The listing builds one solid part. Answer for the finished solid, in the listing's coordinates (mm). A direction names the side the tool comes from. Give positions to 0.01 mm unless a question says otherwise; leave off trailing zeros. Order: outer loops, then holes, each group sorted by start corner. A loop starts at its lowest first (then second) coordinate and runs counter-clockwise, first axis right, second up. Notation, with made-up numbers: (-25.75, 42) - (-18.75, 42) arc R12 ccw to (-18.75, 65) - close; hole circle Ø1 at (35.25, 12). An arc over 180 degrees is marked (long way). Answer in a Markdown table with one row per item. Add a question column.
```python
from build123d import *

# Parameters (mm, degrees)
BOSS_EXTRUDE1_DEPTH     = 300
SKETCH2_W               = 10
SKETCH2_H               = 10
BOSS_EXTRUDE2_DEPTH     = 2
SKETCH4_R               = 18
SKETCH4_R_2             = 15
SKETCH4_R_3             = 10
BOSS_EXTRUDE3_DEPTH     = 2
SKETCH4_3_R             = 10
CUT_EXTRUDE1_DEPTH      = 2
BOSS_EXTRUDE4_START     = -5
BOSS_EXTRUDE4_OUTLINE_R = 12.5
BOSS_EXTRUDE4_DEPTH     = 3
CUT_EXTRUDE2_START      = -2
CUT_EXTRUDE2_DEPTH      = 2
F_3_0MM_DOWEL_HOLE1_D   = 3
SKETCH8_R               = 2.5
BOSS_EXTRUDE5_DEPTH     = 2
SKETCH9_R               = 5
CUT_EXTRUDE3_DEPTH      = 32
SKETCH10_R              = 2.5
CUT_EXTRUDE4_DEPTH      = 10


# Read off the part's stored shape, not the designer's step: Boss-Extrude4, Cut-Extrude2
with BuildPart() as part:
    # Sketch1 → Boss-Extrude1 (new body)
    with BuildSketch(Plane(origin=(0, 0, 0), x_dir=(0, 0, -1), z_dir=(1, 0, 0))):
        with BuildLine():
            Line((10, 13), (10, -13))
            ThreePointArc((10, -13), (9.414213562, -14.414213562), (8, -15))
            Line((8, -15), (0, -15))
            Line((0, -15), (0, -14))
            Line((0, -14), (7, -14))
            ThreePointArc((7, -14), (8.414213562, -13.414213562), (9, -12))
            Line((9, -12), (9, 12))
            ThreePointArc((9, 12), (8.414213562, 13.414213562), (7, 14))
            Line((7, 14), (0, 14))
            Line((0, 14), (0, 15))
            Line((0, 15), (8, 15))
            ThreePointArc((8, 15), (9.414213562, 14.414213562), (10, 13))
        make_face()
    extrude(amount=BOSS_EXTRUDE1_DEPTH)

    # Sketch2 → Boss-Extrude2 (add)
    with BuildSketch(Plane.XY):
        with Locations((75, 20)):
            Rectangle(SKETCH2_W, SKETCH2_H)
        with Locations((75, -20)):
            Rectangle(SKETCH2_W, SKETCH2_H)
        with Locations((225, 20)):
            Rectangle(SKETCH2_W, SKETCH2_H)
        with Locations((225, -20)):
            Rectangle(SKETCH2_W, SKETCH2_H)
    extrude(amount=-BOSS_EXTRUDE2_DEPTH)

    # Sketch4 → Boss-Extrude3 (add)
    # profile 1 of 2: a face of its own
    with BuildSketch(Plane(origin=(0, 0, -10), x_dir=(-1, 0, 0), z_dir=(0, 0, -1))):
        Circle(SKETCH4_R)
        Circle(SKETCH4_R_2, mode=Mode.SUBTRACT)
    # profile 2 of 2: a face of its own
    with BuildSketch(Plane(origin=(0, 0, -10), x_dir=(-1, 0, 0), z_dir=(0, 0, -1))):
        Circle(SKETCH4_R)
        with Locations(Location((0, 0, 0), (0, 0, 90))):
            Circle(SKETCH4_R_3, mode=Mode.SUBTRACT)
    extrude(amount=-BOSS_EXTRUDE3_DEPTH)

    # Sketch4<3> → Cut-Extrude1 (cut)
    with BuildSketch(Plane(origin=(0, 0, -10), x_dir=(-1, 0, 0), z_dir=(0, 0, -1))):
        with Locations(Location((0, 0, 0), (0, 0, 90))):
            Circle(SKETCH4_3_R)
    extrude(amount=-CUT_EXTRUDE1_DEPTH, mode=Mode.SUBTRACT)

    # Boss-Extrude4 outline → Boss-Extrude4 (add)
    with BuildSketch(Plane(origin=(0, 0, -10), x_dir=(-1, 0, 0), z_dir=(0, 0, -1)).offset(BOSS_EXTRUDE4_START)):
        Circle(BOSS_EXTRUDE4_OUTLINE_R)
        with BuildLine():
            ThreePointArc((-9.682458366, 2.5), (10, 0), (-9.682458366, -2.5))
            Line((-9.682458366, -2.5), (-10.25, -2.5))
            ThreePointArc((-10.25, -2.5), (-11.664213562, -1.914213562), (-12.25, -0.5))
            Line((-12.25, -0.5), (-12.25, 0.5))
            ThreePointArc((-12.25, 0.5), (-11.664213562, 1.914213562), (-10.25, 2.5))
            Line((-10.25, 2.5), (-9.682458366, 2.5))
        make_face(mode=Mode.SUBTRACT)
    extrude(amount=BOSS_EXTRUDE4_DEPTH)

    # Cut-Extrude2 outline → Cut-Extrude2 (cut)
    with BuildSketch(Plane(origin=(0, 0, -10), x_dir=(-1, 0, 0), z_dir=(0, 0, -1)).offset(CUT_EXTRUDE2_START)):
        with BuildLine():
            ThreePointArc((-10.25, 2.5), (-11.664213562, 1.914213562), (-12.25, 0.5))
            Line((-12.25, 0.5), (-12.25, -0.5))
            ThreePointArc((-12.25, -0.5), (-11.664213562, -1.914213562), (-10.25, -2.5))
            Line((-10.25, -2.5), (-9.682458366, -2.5))
            ThreePointArc((-9.682458366, -2.5), (-10, 0), (-9.682458366, 2.5))
            Line((-9.682458366, 2.5), (-10.25, 2.5))
        make_face()
    extrude(amount=CUT_EXTRUDE2_DEPTH, mode=Mode.SUBTRACT)

    # Ø3.0mm Dowel Hole1 (through all)
    with Locations(Plane.XY):
        with Locations((75, 20), (75, -20), (225, 20), (225, -20)):
            Hole(F_3_0MM_DOWEL_HOLE1_D / 2)

    # Sketch8 → Boss-Extrude5 (add)
    with BuildSketch(Plane(origin=(300, 0, 0), x_dir=(0, 0, -1), z_dir=(1, 0, 0))):
        with BuildLine():
            Line((0, -5), (0, -20))
            Line((0, -20), (30, -20))
            Line((30, -20), (30, 20))
            Line((30, 20), (0, 20))
            Line((0, 20), (0, 5))
            ThreePointArc((0, 5), (3.535533906, 3.535533906), (5, 0))
            ThreePointArc((5, 0), (3.535533906, -3.535533906), (0, -5))
        make_face()
        with Locations((23, -13)):
            Circle(SKETCH8_R, mode=Mode.SUBTRACT)
        with Locations((23, 13)):
            Circle(SKETCH8_R, mode=Mode.SUBTRACT)
    extrude(amount=-BOSS_EXTRUDE5_DEPTH)

    # Sketch9 → Cut-Extrude3 (cut)
    with BuildSketch(Plane.XY):
        with Locations((272.348806761, 0)):
            Circle(SKETCH9_R)
    extrude(amount=-CUT_EXTRUDE3_DEPTH, mode=Mode.SUBTRACT)

    # Sketch10 → Cut-Extrude4 (cut)
    with BuildSketch(Plane(origin=(0, 0, -10), x_dir=(-1, 0, 0), z_dir=(0, 0, -1))):
        with Locations(Location((0, 14.25, 0), (0, 0, 90))):
            Circle(SKETCH10_R)
        with Locations(Location((12.340862004, -7.125, 0), (0, 0, 90))):
            Circle(SKETCH10_R)
        with Locations(Location((-12.340862004, -7.125, 0), (0, 0, 90))):
            Circle(SKETCH10_R)
    extrude(amount=-CUT_EXTRUDE4_DEPTH, mode=Mode.SUBTRACT)


solid = part.part
```
(1) Find section B-B, the plane z = -15.5. Write down the section's boundary in (x, y), plus the area to 3 significant figures.
(2) Straight lines are drawn through the part: line 1 (Y direction, x = 299, z = -23); line 2 (Z direction, x = 105, y = 4.5); line 3 (X direction, y = -5.5, z = -1.5). For each, find the intervals that lie inside material, in ascending order.
(3) For faces 4 (the face through (1.15, 12.03, -8.36)), 5 (the face through (154, 0, -9)), 6 (the face through (223.8, -18.8, -2)), 7 (the face through (148, 14, -4)), 8 (the face through (162.9, 14.3, 0)), determine the directions among +Z, -Z, +X, -X, +Y, -Y from which every point of the face is accessible in a straight line to the end or side of a thin tool.
(4) The mould has two halves that part along Y. Classify faces 1 (the face through (-17.99, -0.59, -9.01)), 2 (the face through (150.7, -14.2, 0)), 3 (the face through (10.745, 6.388, -6.479)): +Y half, -Y half, draft (parallel to the pull), parting line (faces both ways), or undercut.
(5) Find section A-A, the plane x = 177.5. Write down the section's boundary in (y, z), plus the area to 3 significant figures.
(6) Each of these flat-tipped pins is pushed along its axis until it touches: P1, Ø3.5, axis at x = 108, z = -4.5, coming from the -Y side; P2, Ø11, axis at x = 7, y = -7, coming from the +Z side; P3, Ø8, axis at y = -14, z = -19, coming from the -X side; P4, Ø3, axis at x = 191.5, y = 18, coming from the -Z side. Where does it stop, or does it pass through?
Answer key:
| question | item | result |
|---|---|---|
| 1 | outline | (298, -20) - (300, -20) - (300, 20) - (298, 20) - close |
| 1 | area | 80.0 mm² |
| 2 | line 1 | -20 to -15.5, -10.5 to 10.5, 15.5 to 20 |
| 2 | line 2 | -10 to -9 |
| 2 | line 3 | 298 to 300 |
| 3 | face 4 | +Z, -Z |
| 3 | face 5 | +Z |
| 3 | face 6 | -Z, -X, -Y |
| 3 | face 7 | +Z, -X |
| 3 | face 8 | +Z, +X, -X, +Y, -Y |
| 4 | face 1 | parting line |
| 4 | face 2 | draft |
| 4 | face 3 | undercut |
| 5 | outline | (-15, -8) arc R2 ccw to (-13, -10) - (13, -10) arc R2 ccw to (15, -8) - (15, 0) - (14, 0) - (14, -7) arc R2 cw to (12, -9) - (-12, -9) arc R2 cw to (-14, -7) - (-14, 0) - (-15, 0) - close |
| 5 | area | 48.0 mm² |
| 6 | P1 | y = -15 |
| 6 | P2 | z = -5 |
| 6 | P3 | x = 298 |
| 6 | P4 | through |
